Input: part model. Units: mm. Frame: model coordinates. A direction names the side the tool comes from. Round coordinates to 2 decimals unless told otherwise and drop trailing zeros. Loops run counter-clockwise (first coordinate to the right, second up) from the corner with the lowest first, then second, coordinate; pieces in that order, holes last. Notation, with made-up numbers: (-33, -5.75) - (-20, -5.75) arc R6 cw to (-20, 5.25) - close; hole circle Ø4 at (6.25, 15). An arc over 180 degrees is marked (long way). One line per question, with ' | ' between items. Start each with the question number.
Item 1: Section A-A, the plane z = 4.75. Return loops of the section in (x, y), plus the area to 3 significant figures.
Item 2: Draft query along X for faces 4 (the face through (10.475, 8.533, 12.325)), 5 (the face through (0, 0, 25)), 6 (the face through (-1.9, 22.26, 12.32)), 7 (the face through (-18.33, -12.77, 12.32)). Return one class per face: pulls with the +X half, pulls with the -X half, needs draft (parallel to the pull), parting line crosses it, or undercut.
Item 3: Material intervals for line 1 along X through (y, z) = (-15, 6); line 2 along X through (y, z) = (-19.5, 7.25); line 3 along Y through (x, z) = (-13.5, 1.75), sorted ascending.
Item 4: Section D-D, the plane x = -6.5. Return loops of the section in (y, z).
Item 5: Set-up query: faces 1 (the face through (0, 0, 0)), 2 (the face through (0, -18, 12)), 3 (the face through (13.028, 12.562, 12.325)). Return all of +Z, -Z, +X, -X, +Y, -Y with unobstructed straight access to the full face (end or side cutting, diameter ignored); none if empty.
Item 6: Section B-B, the plane x = -17. Return loops of the section in (y, z).
Item 7: First-contact query: pin 1 (4 mm diameter, centred on x = -16, z = 3.5, fed in from +Y); pin 2 (7 mm diameter, centred on y = -16, z = 14, fed in from -X); pin 3 (4 mm diameter, centred on x = -9.5, z = 2.5, fed in from -Y); pin 4 (6 mm diameter, centred on x = -1.5, z = 4, fed in from +Y). Flat tips, straight axial feed; report the tip coordinate or a pass-through.
Item 8: Section C-C, the plane y = 6. Return loops of the section in (x, z).
```python
from build123d import *

# Parameters (mm, degrees)
F1_DEPTH = 25


with BuildPart() as f1:
    # F0 (on Top) → F1 (new body)
    with BuildSketch(Plane.XY):
        with BuildLine():
            ThreePointArc((4.365322, -21.90869), (17.27086, -14.169126), (22.339354, 0))
            ThreePointArc((22.339354, 0), (21.578159, 5.78185), (19.346448, 11.169677))
            Line((19.346448, 11.169677), (11.551495, 6.669259))
            Line((11.551495, 6.669259), (9.368834, 10.449739))
            Line((9.368834, 10.449739), (16.790821, 14.734825))
            ThreePointArc((16.790821, 14.734825), (-2.193257, 22.231427), (-19.346448, 11.169677))
            Line((-19.346448, 11.169677), (-11.551495, 6.669259))
            Line((-11.551495, 6.669259), (-13.734156, 2.888779))
            Line((-13.734156, 2.888779), (-21.156143, 7.173865))
            ThreePointArc((-21.156143, 7.173865), (-18.156352, -13.01513), (0, -22.339354))
            Line((0, -22.339354), (0, -13.338517))
            Line((0, -13.338517), (4.365322, -13.338517))
            Line((4.365322, -13.338517), (4.365322, -21.90869))
        make_face()
    extrude(amount=F1_DEPTH)


solid = f1.part
```
Return value:
1) outline: (-21.16, 7.17) arc R22.34 ccw to (0, -22.34) - (0, -13.34) - (4.37, -13.34) - (4.37, -21.91) arc R22.34 ccw to (19.35, 11.17) - (11.55, 6.67) - (9.37, 10.45) - (16.79, 14.73) arc R22.34 ccw to (-19.35, 11.17) - (-11.55, 6.67) - (-13.73, 2.89) - close | area: 1,450 mm2
2) face 4: undercut | face 5: needs draft | face 6: parting line crosses it | face 7: pulls with the -X half
3) line 1: -16.55 to 0, 4.37 to 16.55 | line 2: -10.9 to 0, 4.37 to 10.9 | line 3: -17.8 to 3.29, 7.79 to 17.8
4) outline: (-21.37, 0) - (21.37, 0) - (21.37, 25) - (-21.37, 25) - close
5) face 1: -Z, +X, -X, +Y, -Y | face 2: +Z, -Z, -Y | face 3: +Z, -Z
6) outline: (-14.49, 0) - (4.77, 0) - (4.77, 25) - (-14.49, 25) - close; (9.81, 0) - (14.49, 0) - (14.49, 25) - (9.81, 25) - close
7) pin 1: y = 17.41 | pin 2: x = -18.51 | pin 3: y = -21.04 | pin 4: y = 22.34
8) outline: (-21.52, 0) - (-19.12, 0) - (-19.12, 25) - (-21.52, 25) - close; (-11.94, 0) - (21.52, 0) - (21.52, 25) - (-11.94, 25) - close
